Verification items for the finished model (mm, model axes). Face numbers are marked on the shaded views. Give positions to 0.01 mm unless a question says otherwise; leave off trailing zeros. Order: outer loops, then holes, each group sorted by start corner. A loop starts at its lowest first (then second) coordinate and runs counter-clockwise, first axis right, second up.
(1) Sectioned sample at D-D on x = 20. Record the cut outline in (y, z), plus the area to 3 significant figures.
(2) Mould release check, pull along Y, two halves, no side actions. Record for the marked faces 1, 2 and 3: pulls with the +Y half, pulls with the -Y half, needs draft (parallel to the pull), parting line crosses it, or undercut.
(3) Sectioned sample at B-B on y = -17. Record the cut outline in (x, z).
(4) Gauge pin test, flat end, axial feed: pin 1 (1 mm diameter, centred on x = 21.5, z = 16, fed in from +Y). Record the tip position at first contact, or that the pin passes through.
(5) Scan lines: L1, parallel to X at y = -8.5, z = 4; L2, parallel to X at y = -8.25, z = 10; L3, parallel to Y at x = 12, z = 15. Record each from-to range of solid material in increasing order.
(6) Sectioned sample at A-A on x = 2.5. Record the cut outline in (y, z), plus the area to 3 significant figures.
(7) Sectioned sample at C-C on z = 8.75. Record the cut outline in (x, y).
```python
from build123d import *

# Parameters (mm, degrees)
F0_W     = 50
F0_H     = 20
F1_DEPTH = 25
F2_R     = 5
F3_SIZE  = 5
F4_R     = 5.978128
F5_DEPTH = 25


with BuildPart() as f1:
    # F0 (on Front) → F1 (new body)
    with BuildSketch(Plane.XZ):
        with Locations((10.46083, 8.981205)):
            Rectangle(F0_W, F0_H)
    extrude(amount=F1_DEPTH)

    # F2
    f2_edges = [f1.edges().sort_by_distance(p)[0] for p in [
        (10.46083, -25, 18.981205),
    ]]
    fillet(f2_edges, radius=F2_R)

    # F3
    f3_edges = [f1.edges().sort_by_distance(p)[0] for p in [
        (10.46083, 0, 18.981205),
    ]]
    chamfer(f3_edges, length=F3_SIZE)

    # F4 (on face) → F5 (cut)
    with BuildSketch(Plane.XY.offset(18.981205)):
        with Locations((6.721196, -12.210171)):
            Circle(F4_R)
    extrude(amount=-F5_DEPTH, mode=Mode.SUBTRACT)


solid = f1.part
```
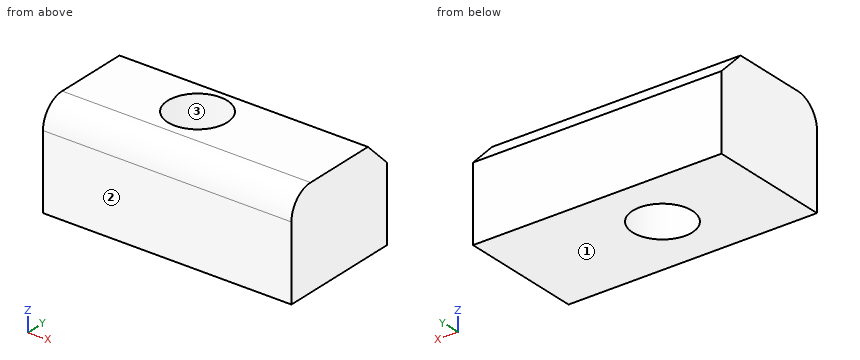
Ans:
1. outline: (-25, -1.02) - (0, -1.02) - (0, 13.98) - (-5, 18.98) - (-20, 18.98) arc R5 ccw to (-25, 13.98) - close
1. area: 482 mm2
2. face 1: needs draft
2. face 2: pulls with the -Y half
2. face 3: undercut
3. outline: (-14.54, -1.02) - (3.14, -1.02) - (3.14, 18.98) - (-14.54, 18.98) - close; (10.3, -1.02) - (35.46, -1.02) - (35.46, 18.98) - (10.3, 18.98) - close
4. pin 1: stops at y = -1.52
5. L1: x = -14.54 to 2.03, 11.41 to 35.46
5. L2: x = -14.54 to 2.24, 11.2 to 35.46
5. L3: y = -24.9 to -15.02, -9.4 to -1.02
6. outline: (-25, -1.02) - (-16.44, -1.02) - (-16.44, 18.98) - (-20, 18.98) arc R5 ccw to (-25, 13.98) - close; (-7.98, -1.02) - (0, -1.02) - (0, 13.98) - (-5, 18.98) - (-7.98, 18.98) - close
6. area: 313 mm2
7. outline: (-14.54, -25) - (35.46, -25) - (35.46, 0) - (-14.54, 0) - close; hole circle Ø11.96 at (6.72, -12.21)
